Build history of the part. All positions in model axes, mm. Coordinates: 2 decimals unless noted, no trailing zeros. Order: outer loops, then holes, each group sorted by start corner. A loop starts at its lowest first (then second) coordinate and runs counter-clockwise, first axis right, second up. Notation, with made-up numbers: (7, 60.5) - (19, 60.5) arc R10 ccw to (19, 76.5) - close; hole circle Ø2 at (58, -31.75). An arc over 180 degrees is marked (long way). Write each question's results on one line, items separated by ' | '.
from build123d import *

# Parameters (mm, degrees)
BOSS_EXTRUDE1_DEPTH = 6
FILLET1_R           = 20
SKETCH9_R           = 1.7
CUT_EXTRUDE7_DEPTH  = 70
SKETCH10_R          = 1.7
CUT_EXTRUDE8_DEPTH  = 10
CUT_EXTRUDE9_DEPTH  = 10
SKETCH12_R          = 2.2
CUT_EXTRUDE10_DEPTH = 10


with BuildPart() as part:
    # Sketch1 → Boss-Extrude1 (new body)
    with BuildSketch(Plane.XY):
        Polygon((80, 138.564064606), (-80, 138.564064606), (-160, 0), (-80, -138.564064606), (80, -138.564064606), (160, 0), align=None)
    extrude(amount=BOSS_EXTRUDE1_DEPTH)

    # Fillet1
    fillet1_edges = [part.edges().sort_by_distance(p)[0] for p in [
        (160, 0, 3),
        (80, -138.564064606, 3),
        (-80, -138.564064606, 3),
        (-160, 0, 3),
        (-80, 138.564064606, 3),
        (80, 138.564064606, 3),
    ]]
    fillet(fillet1_edges, radius=FILLET1_R)

    # Sketch9 → Cut-Extrude7 (cut)
    with BuildSketch(Plane.XY.offset(6)):
        with Locations((-75.381197846, -130.564064606)):
            Circle(SKETCH9_R)
        with Locations((75.381197846, -130.564064606)):
            Circle(SKETCH9_R)
        with Locations((-75.381197846, 130.564064606)):
            Circle(SKETCH9_R)
        with Locations((-150.762395693, 0)):
            Circle(SKETCH9_R)
        with Locations((150.762395693, 0)):
            Circle(SKETCH9_R)
        with Locations((75.381197846, 130.564064606)):
            Circle(SKETCH9_R)
    extrude(amount=-CUT_EXTRUDE7_DEPTH, mode=Mode.SUBTRACT)

    # Sketch10 → Cut-Extrude8 (cut)
    with BuildSketch(Plane.XY.offset(6)):
        with Locations((-88.437426954, -5)):
            Circle(SKETCH10_R)
        with Locations((-21.437426954, -5)):
            Circle(SKETCH10_R)
        with Locations((-14.937426954, -87)):
            Circle(SKETCH10_R)
        with Locations((-94.937426954, -87)):
            Circle(SKETCH10_R)
    extrude(amount=-CUT_EXTRUDE8_DEPTH, mode=Mode.SUBTRACT)

    # Sketch11 → Cut-Extrude9 (cut)
    with BuildSketch(Plane.XY.offset(6)):
        with BuildLine():
            Line((48.25, 37.808388537), (48.25, 27.808388537))
            ThreePointArc((48.25, 27.808388537), (46.5, 26.058388537), (44.75, 27.808388537))
            Line((44.75, 27.808388537), (44.75, 37.808388537))
            ThreePointArc((44.75, 37.808388537), (46.5, 39.558388537), (48.25, 37.808388537))
        make_face()
        with BuildLine():
            Line((48.25, -38.75), (48.25, -28.75))
            ThreePointArc((48.25, -28.75), (46.5, -27), (44.75, -28.75))
            Line((44.75, -28.75), (44.75, -38.75))
            ThreePointArc((44.75, -38.75), (46.5, -40.5), (48.25, -38.75))
        make_face()
    extrude(amount=-CUT_EXTRUDE9_DEPTH, mode=Mode.SUBTRACT)

    # Sketch12 → Cut-Extrude10 (cut)
    with BuildSketch(Plane.XY.offset(6)):
        with Locations((0, -113.564064606)):
            Circle(SKETCH12_R)
        with Locations((-98.349364905, 56.782032303)):
            Circle(SKETCH12_R)
        with Locations((98.349364905, 56.782032303)):
            Circle(SKETCH12_R)
    extrude(amount=-CUT_EXTRUDE10_DEPTH, mode=Mode.SUBTRACT)


solid = part.part
1. Band-saw the part on A-A on y = -34.5. Give the cut face in (x, z).
Solved:
outline: (-140.08, 0) - (44.75, 0) - (44.75, 6) - (-140.08, 6) - close; (48.25, 0) - (140.08, 0) - (140.08, 6) - (48.25, 6) - close
2. Drop flat-ended pins along their axis: pin 1 Ø3 at (y, z) = (-35.5, 4) entering from -X; pin 2 Ø2.5 at (x, y) = (-75.38, -130.56) entering from -Z; pin 3 Ø1.8 at (y, z) = (32.5, 2) entering from -X; pin 4 Ø1 at (y, z) = (0.5, 2.5) entering from -X. Give the stop position or say it passes through.
Solved:
pin 1: stops at x = -140.37 | pin 2: passes through | pin 3: stops at x = -141.76 | pin 4: stops at x = -156.91
3. Band-saw the part on B-B on z = 4.75. Give the number of separate pieces and of enclosed holes in the cut face, then the cut area to 3 significant figures.
Solved:
separate pieces: 1 | enclosed holes: 15 | area: 66,200 mm2
4. Probe line 1 (Y direction, x = 0, z = 2.15); line 2 (X direction, y = -5.5, z = 5.65); line 3 (X direction, y = 57, z = 3.6). List the from-to ranges inside material, lowest first.
Solved:
line 1: y = -138.56 to -115.76, -111.36 to 138.56 | line 2: x = -156.13 to -90.06, -86.81 to -23.06, -19.81 to 156.13 | line 3: x = -127.09 to -100.54, -96.16 to 96.16, 100.54 to 127.09
5. Band-saw the part on D-D on y = 79. Give the cut face in (x, z).
Solved:
outline: (-114.39, 0) - (114.39, 0) - (114.39, 6) - (-114.39, 6) - close
6. Band-saw the part on C-C on y = -64.5. Give the cut face in (x, z).
Solved:
outline: (-122.76, 0) - (122.76, 0) - (122.76, 6) - (-122.76, 6) - close
